```python
from build123d import *

# Parameters (mm, degrees)
BOSS_EXTRUDE3_DEPTH = 7.8
SKETCH2_R           = 2.4
CUT_EXTRUDE9_DEPTH  = 7.8
SKETCH3_R           = 3.05
CUT_EXTRUDE10_DEPTH = 0.8
SKETCH4_R           = 3.05
CUT_EXTRUDE11_DEPTH = 0.8


with BuildPart() as part:
    # Sketch1 → Boss-Extrude3 (new body)
    with BuildSketch(Plane(origin=(0, 0, 0), x_dir=(1, 0, 0), z_dir=(0, 1, 0))):
        with BuildLine():
            Line((-12.3, 3.7), (16, 3.7))
            ThreePointArc((16, 3.7), (19.7, 0), (16, -3.7))
            Line((16, -3.7), (-16, -3.7))
            ThreePointArc((-16, -3.7), (-18.61629509, -2.61629509), (-19.7, 0))
            Line((-19.7, 0), (-19.7, 16))
            ThreePointArc((-19.7, 16), (-16, 19.7), (-12.3, 16))
            Line((-12.3, 16), (-12.3, 3.7))
        make_face()
    extrude(amount=BOSS_EXTRUDE3_DEPTH)

    # Sketch2 → Cut-Extrude9 (cut)
    with BuildSketch(Plane(origin=(0, 7.8, 0), x_dir=(1, 0, 0), z_dir=(0, 1, 0))):
        Circle(SKETCH2_R)
        with Locations((8, 0)):
            Circle(SKETCH2_R)
        with Locations((16, 0)):
            Circle(SKETCH2_R)
        with Locations((-16, 0)):
            Circle(SKETCH2_R)
        with Locations((-8, 0)):
            Circle(SKETCH2_R)
        with Locations((-16, 16)):
            Circle(SKETCH2_R)
        with Locations((-16, 8)):
            Circle(SKETCH2_R)
    extrude(amount=-CUT_EXTRUDE9_DEPTH, mode=Mode.SUBTRACT)

    # Sketch3 → Cut-Extrude10 (cut)
    with BuildSketch(Plane(origin=(0, 7.8, 0), x_dir=(1, 0, 0), z_dir=(0, 1, 0))):
        Circle(SKETCH3_R)
        with Locations((8, 0)):
            Circle(SKETCH3_R)
        with Locations((16, 0)):
            Circle(SKETCH3_R)
        with Locations((-16, 0)):
            Circle(SKETCH3_R)
        with Locations((-8, 0)):
            Circle(SKETCH3_R)
        with Locations((-16, 8)):
            Circle(SKETCH3_R)
        with Locations((-16, 16)):
            Circle(SKETCH3_R)
    extrude(amount=-CUT_EXTRUDE10_DEPTH, mode=Mode.SUBTRACT)

    # Sketch4 → Cut-Extrude11 (cut)
    with BuildSketch(Plane.XZ):
        Circle(SKETCH4_R)
        with Locations((8, 0)):
            Circle(SKETCH4_R)
        with Locations((16, 0)):
            Circle(SKETCH4_R)
        with Locations((-16, 0)):
            Circle(SKETCH4_R)
        with Locations((-8, 0)):
            Circle(SKETCH4_R)
        with Locations((-16, -8)):
            Circle(SKETCH4_R)
        with Locations((-16, -16)):
            Circle(SKETCH4_R)
    extrude(amount=-CUT_EXTRUDE11_DEPTH, mode=Mode.SUBTRACT)


solid = part.part
```
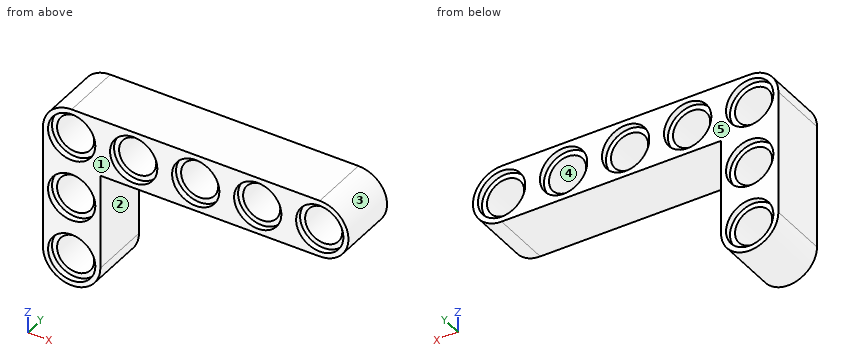
Source: CAD feature listing. Evaluate the final solid. Frame: model axes, mm. Face numbers are marked on the shaded views. A direction names the side the tool comes from. Round coordinates to 2 decimals unless told otherwise and drop trailing zeros. Write each loop counter-clockwise with the first axis right and the second up, starting at its lowest first coordinate (ties: lowest second). Pieces come first, ordered by that corner, then holes. Notation, with made-up numbers: M -13.75,44.25 L 39.25,44.25 A26 ccw 39.25,69.25 Z; hole C 27.5,-10.75 d3. An arc over 180 degrees is marked long. Use CSV: the item, a comma, the result in double quotes. Start each with the question number.
Q1. Cut plane D-D on z = -1.5. Count the separate pieces of the cut face and the enclosed holes in it, plus the area to 3 significant figures.
Q2. Cut plane A-A on y = 1.75. Output: boundary loops of the cut face in (x, z), plus the area to 3 significant figures.
Q3. First-contact query: P1, Ø4.5, axis at x = -16, z = -8, coming from the +Y side; P2, Ø1.5, axis at x = 2.5, y = 3.5, coming from the -Z side; P3, Ø5.5, axis at x = -8, z = 0, coming from the -Y side; P4, Ø1, axis at y = 2, z = -4.5, coming from the +X side. Flat tips, straight axial feed; report the tip coordinate or a pass-through.
Q4. Access query for the marked faces 1 and 2. Directions: +Z, -Z, +X, -X, +Y, -Y. A direction counts if a zero-diameter tool reaches every point of the face in a straight line with its end or side. Return the directions, or none.
Q5. Line query: line 1 (X direction, y = 2.5, z = 0); line 2 (Z direction, x = -16, y = 0.35); line 3 (X direction, y = 7.45, z = 0). Output: solid intervals per line, ascending. Write a range as from..to.
Q6. Pull-direction query (Z, two-part tool) for the marked faces 3, 4 and 5; classes: +Z half, -Z half, draft (parallel to the pull), parting line (faces both ways), or undercut.
Q7. Cut plane C-C on z = -15.25. Output: boundary loops of the cut face in (x, y).
Q8. Cut plane B-B on x = 0.5. Output: boundary loops of the cut face in (y, z).
Results found:
1,separate pieces,"6"
1,enclosed holes,"0"
1,area,"146 mm^2"
2,outline,"M -19.7,-16 A3.7 ccw -12.3,-16 L -12.3,-3.7 L 16,-3.7 A3.7 ccw 16,3.7 L -16,3.7 A3.7 ccw -19.7,0 Z; hole C -16,-16 d4.8; hole C -16,-8 d4.8; hole C -16,0 d4.8; hole C -8,0 d4.8; hole C 0,0 d4.8; hole C 8,0 d4.8; hole C 16,0 d4.8"
2,area,"269 mm^2"
3,P1,"through"
3,P2,"z = -3.7"
3,P3,"y = 0.8"
3,P4,"x = -12.3"
4,face 1,"+Z, -Z, +X, -X, -Y"
4,face 2,"-Z, +X, +Y, -Y"
5,line 1,"-19.7..-18.4, -13.6..-10.4, -5.6..-2.4, 2.4..5.6, 10.4..13.6, 18.4..19.7"
5,line 2,"-19.7..-19.05, -12.95..-11.05, -4.95..-3.05, 3.05..3.7"
5,line 3,"-19.7..-19.05, -12.95..-11.05, -4.95..-3.05, 3.05..4.95, 11.05..12.95, 19.05..19.7"
6,face 3,"parting line"
6,face 4,"undercut"
6,face 5,"draft"
7,outline,"M -19.7,0 L -18.96,0 L -18.96,0.8 L -18.28,0.8 L -18.28,7 L -18.96,7 L -18.96,7.8 L -19.7,7.8 Z; M -13.72,0.8 L -13.04,0.8 L -13.04,0 L -12.3,0 L -12.3,7.8 L -13.04,7.8 L -13.04,7 L -13.72,7 Z"
8,outline,"M 0,-3.7 L 7.8,-3.7 L 7.8,-3.01 L 7,-3.01 L 7,-2.35 L 0.8,-2.35 L 0.8,-3.01 L 0,-3.01 Z; M 0,3.01 L 0.8,3.01 L 0.8,2.35 L 7,2.35 L 7,3.01 L 7.8,3.01 L 7.8,3.7 L 0,3.7 Z"
